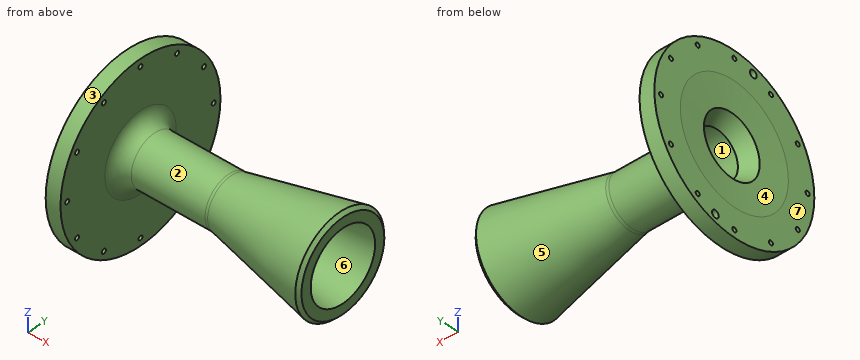
```python
from build123d import *

# Parameters (mm, degrees)
FLANGE_HOLES_D     = 2.8702
FLANGE_HOLES_DEPTH = 9.525
DOWEL_HOLES_D      = 4.7625
DOWEL_HOLES_DEPTH  = 6.35
DOWEL_HOLES_TIP    = 1.430799349
FILLET1_R          = 8.89
CHAMFER1_SIZE2     = 2.54
CHAMFER1_SIZE      = 2.141545552


with BuildPart() as part:
    # Sketch2 → Main Structure (revolve)
    with BuildSketch(Plane.XY):
        Polygon((0, 20.583496156), (0, 56.388), (9.525, 56.388), (9.525, 16.256), (66.806461084, 16.256), (139.7, 31.75), (139.7, 22.7076), (60.325, 12.720781818), (60.325, 14.351), (10.795, 14.351), align=None)
    revolve(axis=Axis((0, 0, 0), (1, 0, 0)))

    # Flange Holes
    with Locations(Plane.ZY):
        with Locations((0, -51.6255), (-25.81275, -44.708994483), (-44.708994483, -25.81275), (-51.6255, 0), (-44.708994483, 25.81275), (-25.81275, 44.708994483), (0, 51.6255), (25.81275, 44.708994483), (44.708994483, 25.81275), (51.6255, 0), (44.708994483, -25.81275), (25.81275, -44.708994483)):
            Hole(FLANGE_HOLES_D / 2, depth=FLANGE_HOLES_DEPTH)

    # Dowel Holes
    with Locations(Plane.ZY):
        with Locations((49.866403745, -13.361662613), (-49.866403745, 13.361662613)):
            Hole(DOWEL_HOLES_D / 2, depth=DOWEL_HOLES_DEPTH)
            with Locations((0, 0, -(DOWEL_HOLES_DEPTH + DOWEL_HOLES_TIP / 2))):  # 118° drill point
                Cone(0, DOWEL_HOLES_D / 2, DOWEL_HOLES_TIP, mode=Mode.SUBTRACT)

    # Fillet1
    fillet1_edges = [part.edges().sort_by_distance(p)[0] for p in [
        (66.806461084, -16.256, 0),
        (9.525, -16.256, 0),
    ]]
    fillet(fillet1_edges, radius=FILLET1_R)

    # Sketch13 → Cut-Revolve1 (revolve, cut)
    with BuildSketch(Plane(origin=(0, 0, 0), x_dir=(1, 0, 0), z_dir=(0, 1, 0))):
        Polygon((0, 38.1), (3.33331808, 0), (0, 0), align=None)
    revolve(axis=Axis((3.33331808, 0, 0), (-1, 0, 0)), mode=Mode.SUBTRACT)

    # Chamfer1
    chamfer1_edges = [part.edges().sort_by_distance(p)[0] for p in [
        (139.7, -31.75, 0),
    ]]
    chamfer(chamfer1_edges, length=CHAMFER1_SIZE, length2=CHAMFER1_SIZE2)


solid = part.part
```
Could you check a few things on this model? Use its own coordinates, in mm. Face numbers are marked on the shaded views. A direction names the side the tool comes from. Coordinates: 2 decimals unless noted, no trailing zeros. Loops run counter-clockwise (first coordinate to the right, second up) from the corner with the lowest first, then second, coordinate; pieces in that order, holes last.
1) Will these pins go through, and if not, where does the flat tip stop? pin 1 Ø7.5 at (y, z) = (13.36, -49.87) entering from -X; pin 2 Ø3.5 at (y, z) = (-44.71, 25.81) entering from +X (3 decimals); pin 3 Ø12 at (x, z) = (101, 21) entering from -Y; pin 4 Ø8 at (x, y) = (91, 22) entering from +Z.
Reported:
pin 1: stops at x = 0
pin 2: stops at x = 9.525
pin 3: stops at y = -18.39
pin 4: stops at z = 11.77
2) Imagine slicing it at C-C (x = 96.5). List the corners of the cut face in (y, z) for me, and give its area (3 significant figures).
Reported:
outline: circle Ø45.14 at (0, 0); hole circle Ø34.54 at (0, 0)
area: 663 mm2
3) Thinking about a two-plate mould opening in Z: for the marked faces 4, 5, 6 and 7, which applies, released by +Z, released by -Z, zero draft, split by the parting line, or undercut?
Reported:
face 4: undercut
face 5: split by the parting line
face 6: undercut
face 7: zero draft
4) Imagine slicing it at B-B (z = -40). List the corners of the cut face in (x, y) for me (3 decimals).
Reported:
outline: (0, -39.744) - (9.525, -39.744) - (9.525, 39.744) - (0, 39.744) - close
5) Which directions (+Z, -Z, +X, -X, +Y, -Y) give clear straight access to the entire face, cutting with the end or side of a thin tool? Please do the marked faces 1, 2 and 3.
Reported:
face 1: -X
face 2: none
face 3: +X, -X
6) Imagine slicing it at A-A (x = 31.5). List the corners of the cut face in (y, z) for me.
Reported:
outline: circle Ø32.51 at (0, 0); hole circle Ø28.7 at (0, 0)
7) Imagine slicing it at D-D (z = 41). List the corners of the cut face in (x, y) for me (3 decimals), and give its area (3 significant figures).
Reported:
outline: (0, -38.712) - (9.525, -38.712) - (9.525, 38.712) - (0, 38.712) - close
area: 737 mm2
8) Please list where these lines run through material, in increasing order: line 1 along X through (y, z) = (-5.5, 47.5) (3 decimals); line 2 along Z through (x, y) = (116, 13); line 3 along Z through (x, y) = (107.5, -11.5).
Reported:
line 1: x = 0 to 9.525
line 2: z = -23.34 to -14.84, 14.84 to 23.34
line 3: z = -22.09 to -14.69, 14.69 to 22.09
